from build123d import *

# Parameters (mm, degrees)
F1_DEPTH = 50.8
F3_DEPTH = 25.4


# Not quite as in the source:
# - a feature names something its author has since deleted; it is built from what else it names


with BuildPart() as f1:
    # F0 (on Front) → F1 (new body)
    with BuildSketch(Plane.XZ):
        with BuildLine():
            Line((-37.0038875103, 50.8), (-62.4038875103, 50.8))
            Line((-62.4038875103, 50.8), (-62.4038875103, 25.4))
            Line((-62.4038875103, 25.4), (-48.6759059699, 25.4))
            ThreePointArc((-48.6759059699, 25.4), (-45.2572509132, 33.6533634029), (-37.0038875103, 37.0720184596))
            Line((-37.0038875103, 37.0720184596), (-37.0038875103, 50.8))
        make_face()
        with BuildLine():
            Line((-48.6759059699, 25.4), (-62.4038875103, 25.4))
            Line((-62.4038875103, 25.4), (-62.4038875103, 0))
            Line((-62.4038875103, 0), (-37.0038875103, 0))
            Line((-37.0038875103, 0), (-37.0038875103, 13.7279815404))
            ThreePointArc((-37.0038875103, 13.7279815404), (-45.2572509132, 17.1466365971), (-48.6759059699, 25.4))
        make_face()
        with BuildLine():
            Line((-11.6038875103, 50.8), (-37.0038875103, 50.8))
            Line((-37.0038875103, 50.8), (-37.0038875103, 37.0720184596))
            ThreePointArc((-37.0038875103, 37.0720184596), (-28.7505241074, 33.6533634029), (-25.3318690507, 25.4))
            Line((-25.3318690507, 25.4), (-11.6038875103, 25.4))
            Line((-11.6038875103, 25.4), (-11.6038875103, 50.8))
        make_face()
        with BuildLine():
            Line((-37.0038875103, 13.7279815404), (-37.0038875103, 0))
            Line((-37.0038875103, 0), (-11.6038875103, 0))
            Line((-11.6038875103, 0), (-11.6038875103, 25.4))
            Line((-11.6038875103, 25.4), (-25.3318690507, 25.4))
            ThreePointArc((-25.3318690507, 25.4), (-28.7505241074, 17.1466365971), (-37.0038875103, 13.7279815404))
        make_face()
    extrude(amount=F1_DEPTH)

    # F2 (on face) → F3 (join)
    with BuildSketch(Plane(origin=(-62.4038875103, 0, 0), x_dir=(0, -1, 0), z_dir=(-1, 0, 0))):
        Polygon((16.7379435152, 28.2901115716), (17.1399507672, 13.7242572382), (34.1606251895, 13.7242572382), (34.1606251895, 28.2901115716), align=None)
    extrude(amount=F3_DEPTH)


solid = f1.part
Work out the finished part from the listing and answer in its coordinate system (mm). A direction names the side the tool comes from. Give positions to 0.01 mm unless a question says otherwise; leave off trailing zeros. Write each loop counter-clockwise with the first axis right and the second up, starting at its lowest first coordinate (ties: lowest second). Pieces come first, ordered by that corner, then holes. Notation, with made-up numbers: (29.25, 43.5) - (43.25, 43.5) arc R29 cw to (43.25, 68.5) - close; hole circle Ø2 at (-5, 53.5). An arc over 180 degrees is marked (long way). One line per item, written item: value. Start each with the question number.
1. Given pin 1 (8 mm diameter, centred on x = -72.5, z = 34, fed in from -Y); pin 2 (11.5 mm diameter, centred on x = -69, z = 21.5, fed in from -Y); pin 3 (5 mm diameter, centred on x = -73.5, y = -29, fed in from +Z); pin 4 (8.5 mm diameter, centred on x = -79.5, y = -23.5, fed in from -Z), each flat-ended and moving along its own axis, determine where each tip first touches the part or whether it passes through.
2. For faces 1 (the flat face through (-75, -26, 28.29)), 2 (the flat face through (-43, 0, 14)), 3 (the flat face through (-75, -34.161, 21)), 4 (the flat face through (-75, -26, 13.724)), 5 (the flat face through (-37, -25, 0)), determine the directions among +Z, -Z, +X, -X, +Y, -Y from which every point of the face is accessible in a straight line to the end or side of a thin tool.
3. Find section B-B (z = 18). Write down the section's boundary in (x, y).
4. Find section D-D (y = -19). Write down the section's boundary in (x, z).
5. For a pull along X with two mould halves and no side action, classify faces 6 (the flat face through (-11.604, -25, 25)), 7 (the flat face through (-43, -50.8, 14)), 8 (the flat face through (-87.804, -25, 21)) as +X half, -X half, draft (parallel to the pull), parting line (faces both ways), or undercut.
6. Find section A-A (y = -44). Write down the section's boundary in (x, z), then the cut area to 3 significant figures.
7. Find section C-C (x = -42). Write down the section's boundary in (y, z).
8. Consider probe 1 along X at (y, z) = (-17.5, 25); probe 2 along Z at (x, y) = (-33, -8); probe 3 along X at (y, z) = (-28.5, 31). Determine where each line is inside the solid, lowest interval first.
Geometry results:
1. pin 1: through
1. pin 2: y = -34.16
1. pin 3: z = 28.29
1. pin 4: z = 13.72
2. face 1: +Z, -X, +Y, -Y
2. face 2: +Z, -Z, +X, -X, +Y
2. face 3: +Z, -Z, -X, -Y
2. face 4: -Z, -X, +Y, -Y
2. face 5: -Z, +X, -X, +Y, -Y
3. outline: (-87.8, -34.16) - (-62.4, -34.16) - (-62.4, -50.8) - (-46.03, -50.8) - (-46.03, 0) - (-62.4, 0) - (-62.4, -17.02) - (-87.8, -17.02) - close; (-27.98, -50.8) - (-11.6, -50.8) - (-11.6, 0) - (-27.98, 0) - close
4. outline: (-87.8, 13.72) - (-62.4, 13.72) - (-62.4, 0) - (-11.6, 0) - (-11.6, 50.8) - (-62.4, 50.8) - (-62.4, 28.29) - (-87.8, 28.29) - close; hole circle Ø23.34 at (-37, 25.4)
5. face 6: +X half
5. face 7: draft
5. face 8: -X half
6. outline: (-62.4, 0) - (-11.6, 0) - (-11.6, 50.8) - (-62.4, 50.8) - close; hole circle Ø23.34 at (-37, 25.4)
6. area: 2,150 mm2
7. outline: (-50.8, 0) - (0, 0) - (0, 14.85) - (-50.8, 14.85) - close; (-50.8, 35.95) - (0, 35.95) - (0, 50.8) - (-50.8, 50.8) - close
8. probe 1: -87.8 to -48.67, -25.34 to -11.6
8. probe 2: 0 to 14.44, 36.36 to 50.8
8. probe 3: -62.4 to -47.24, -26.76 to -11.6
